```python
from build123d import *

# Parameters (mm, degrees)
SKETCH_1_W          = 20
SKETCH_1_H          = 12
EXTRUDE_1_DEPTH     = 2.5
SKETCH_1_8_R        = 0.5
CUT_EXTRUDE_1_DEPTH = 3
SKETCH_1_9_R        = 2.6
SKETCH_1_9_R_2      = 1.25
CUT_EXTRUDE_3_DEPTH = 2.5
EXTRUDE_START       = 2.5
SKETCH_1_10_W       = 20
SKETCH_1_10_H       = 12
SKETCH_1_10_R       = 3.5
EXTRUDE_2_DEPTH     = 5
SKETCH_2_R          = 0.7
CUT_EXTRUDE_4_DEPTH = 25.5
CUT_EXTRUDE_START   = -7.5
SKETCH_2_3_R        = 1
CUT_EXTRUDE_5_DEPTH = 5.5
SKETCH_2_6_R        = 0.3
CUT_EXTRUDE_6_DEPTH = 6


with BuildPart() as part:
    # 草图1 → 凸台-拉伸1 (new body)
    with BuildSketch(Plane(origin=(0, 0, 0), x_dir=(1, 0, 0), z_dir=(0, 1, 0))):
        with Locations((10, -6)):
            Rectangle(SKETCH_1_W, SKETCH_1_H)
    extrude(amount=EXTRUDE_1_DEPTH)

    # 草图1<8> → 切除-拉伸1 (cut)
    with BuildSketch(Plane(origin=(0, 0, 0), x_dir=(1, 0, 0), z_dir=(0, 1, 0))):
        with Locations(Location((7.678736094, -8.970584613, 0), (0, 0, 90))):
            Circle(SKETCH_1_8_R)
    extrude(amount=CUT_EXTRUDE_1_DEPTH, mode=Mode.SUBTRACT)

    # 草图1<9> → 切除-拉伸3 (cut)
    with BuildSketch(Plane(origin=(0, 0, 0), x_dir=(1, 0, 0), z_dir=(0, 1, 0))):
        with Locations(Location((9.847079862, -3.807418404, 0), (0, 0, 270))):
            Circle(SKETCH_1_9_R)
        with Locations(Location((15, -6, 0), (0, 0, 270))):
            Circle(SKETCH_1_9_R_2)
    extrude(amount=CUT_EXTRUDE_3_DEPTH, mode=Mode.SUBTRACT)

    # 草图1<10> → 凸台-拉伸2 (add)
    with BuildSketch(Plane(origin=(0, 0, 0), x_dir=(1, 0, 0), z_dir=(0, 1, 0)).offset(EXTRUDE_START)):
        with Locations((10, -6)):
            Rectangle(SKETCH_1_10_W, SKETCH_1_10_H)
        with Locations(Location((15, -6, 0), (0, 0, 90))):
            Circle(SKETCH_1_10_R, mode=Mode.SUBTRACT)
    extrude(amount=EXTRUDE_2_DEPTH)

    # 草图2 → 切除-拉伸4 (cut, through all)
    with BuildSketch(Plane.XZ):
        with Locations(Location((15, 10.9, 0), (0, 0, 270))):
            Circle(SKETCH_2_R)
        with Locations(Location((1.5, 6, 0), (0, 0, 270))):
            Circle(SKETCH_2_R)
        with Locations(Location((16.5, 1.1, 0), (0, 0, 270))):
            Circle(SKETCH_2_R)
    extrude(amount=-CUT_EXTRUDE_4_DEPTH, mode=Mode.SUBTRACT)

    # 草图2<3> → 切除-拉伸5 (cut)
    with BuildSketch(Plane.XZ.offset(CUT_EXTRUDE_START)):
        with Locations(Location((16.5, 1.1, 0), (0, 0, 90))):
            Circle(SKETCH_2_3_R)
        with Locations(Location((15, 10.9, 0), (0, 0, 90))):
            Circle(SKETCH_2_3_R)
        with Locations(Location((1.5, 6, 0), (0, 0, 90))):
            Circle(SKETCH_2_3_R)
    extrude(amount=CUT_EXTRUDE_5_DEPTH, mode=Mode.SUBTRACT)

    # 草图2<6> → 切除-拉伸6 (cut)
    with BuildSketch(Plane.XZ.offset(CUT_EXTRUDE_START)):
        with Locations(Location((12.8, 11.05, 0), (0, 0, 90))):
            Circle(SKETCH_2_6_R)
        with Locations(Location((17.2, 11.05, 0), (0, 0, 90))):
            Circle(SKETCH_2_6_R)
        with Locations(Location((15, 1.3, 0), (0, 0, 90))):
            Circle(SKETCH_2_6_R)
    extrude(amount=CUT_EXTRUDE_6_DEPTH, mode=Mode.SUBTRACT)


solid = part.part
```
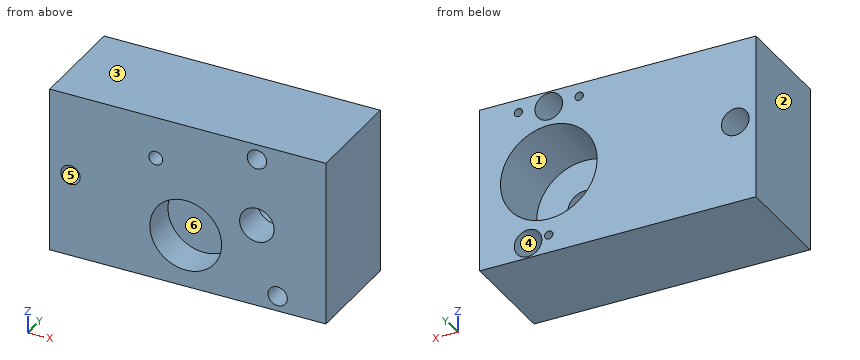
Model file for the job. Use its own axes, mm. Face numbers are marked on the shaded views. A direction names the side the tool comes from. Coordinates: 2 decimals unless noted, no trailing zeros. Loops run counter-clockwise (first coordinate to the right, second up) from the corner with the lowest first, then second, coordinate; pieces in that order, holes last. Notation, with made-up numbers: (-5.75, 45.5) - (25.25, 45.5) arc R24 cw to (25.25, 77.5) - close; hole circle Ø1 at (-0.5, 49.5). An arc over 180 degrees is marked (long way). Answer as a JSON object with one key per item and string values. Group by question number.
(1) Tool access for the marked faces 4, 5 and 6: list every direction of +Z, -Z, +X, -X, +Y, -Y with a clear straight run to the whole face (end or side of a thin tool).
(2) Flat gauge pin, fed straight in: pin 1 (1.8 mm diameter, centred on x = 1.5, z = 6, fed in from +Y). Where does the tip first touch, or does it go through?
(3) Two-plate mould, pull along X, no slides. Class the marked faces 1, 2 and 3: released by +X, released by -X, zero draft, split by the parting line, or undercut.
(4) Cut at D-D (z = 10.5). Give the cut face in (x, y).
(5) Cut at C-C (x = 15). Give the cut face in (y, z).
(6) Probe line 1 along X through (y, z) = (6.05, 6); line 2 along X through (y, z) = (6.25, 5.25); line 3 along X through (y, z) = (1.45, 6). List the from-to ranges inside material, lowest first.
(7) Cut at B-B (y = 4.5). Give the cut face in (x, z), then the cut area to 3 significant figures.
(8) Cut at A-A (x = 1.5). Give the cut face in (y, z), then the cut area to 3 significant figures.
Geometry says:
{
 "1": {"face 4": "+Y", "face 5": "+Y, -Y", "face 6": "-Y"},
 "2": {"pin 1": "stops at y = 2"},
 "3": {"face 1": "undercut", "face 2": "released by -X", "face 3": "zero draft"},
 "4": {"outline": "(0, 0) - (14.43, 0) - (14.43, 2) - (14.08, 2) - (14.08, 7.5) - (0, 7.5) - close; (15.57, 0) - (20, 0) - (20, 7.5) - (15.92, 7.5) - (15.92, 2) - (15.57, 2) - close"},
 "5": {"outline": "(0, 0) - (7.5, 0) - (7.5, 1) - (1.5, 1) - (1.5, 1.6) - (7.5, 1.6) - (7.5, 2.5) - (2.5, 2.5) - (2.5, 4.75) - (0, 4.75) - close; (0, 7.25) - (2.5, 7.25) - (2.5, 9.5) - (7.5, 9.5) - (7.5, 9.9) - (2, 9.9) - (2, 10.2) - (0, 10.2) - close; (0, 11.6) - (2, 11.6) - (2, 11.9) - (7.5, 11.9) - (7.5, 12) - (0, 12) - close"},
 "6": {"line 1": "x = 0 to 0.5, 2.5 to 11.5, 18.5 to 20", "line 2": "x = 0 to 0.84, 2.16 to 11.58, 18.42 to 20", "line 3": "x = 0 to 0.8, 2.2 to 8.45, 11.24 to 13.75, 16.25 to 20"},
 "7": {"outline": "(0, 0) - (20, 0) - (20, 12) - (0, 12) - close; hole circle Ø2 at (1.5, 6); hole circle Ø7 at (15, 6); hole circle Ø0.6 at (12.8, 11.05); hole circle Ø2 at (15, 10.9); hole circle Ø0.6 at (15, 1.3); hole circle Ø2 at (16.5, 1.1); hole circle Ø0.6 at (17.2, 11.05)", "area": "191 mm^2"},
 "8": {"outline": "(0, 0) - (7.5, 0) - (7.5, 5) - (2, 5) - (2, 5.3) - (0, 5.3) - close; (0, 6.7) - (2, 6.7) - (2, 7) - (7.5, 7) - (7.5, 12) - (0, 12) - close", "area": "76.2 mm^2"}
}
